Autodesk Inventor part; units mm, degrees
ref_plane "YZ Plane" through (0, 0, 0) normal (1, 0, 0) x (0, 1, 0)
ref_plane "XZ Plane" through (0, 0, 0) normal (0, 1, 0) x (-1, 0, 0)
ref_plane "XY Plane" through (0, 0, 0) normal (0, 0, 1) x (1, 0, 0)
sketch "Эскиз1" plane through (0, 0, 0) normal (0, 0, 1) x (1, 0, 0)
  line L0 (0, 0) -> (0, -10)
  line L1 (0, -10) -> (4, -10)
  line L2 (4, -10) -> (4, -26)
  line L3 (4, -26) -> (0, -26)
  line L4 (0, -26) -> (0, -29.9118)
  line L5 (0, -29.9118) -> (-1, -29.9118)
  arc A0 (-1, -29.9118) -> (-26.9172, -1) centre (-40, -38.8) ccw
  line L6 (-26.9172, -1) -> (-26.9172, 0)
  line L7 (-26.9172, 0) -> (-26, 0)
  line L8 (-26, 0) -> (-26, 4)
  line L9 (-26, 4) -> (-10, 4)
  line L10 (-10, 4) -> (-10, 0)
  line L11 (-10, 0) -> (0, 0)
  dimension "d0" = 40
  dimension "d1" = 1
  dimension "d3" = 38.8
  dimension "d4" = 4
  dimension "d5" = 40
  dimension "d6" = 16
  dimension "d7" = 10
  dimension "d8" = 16
  dimension "d9" = 10
extrude "Выдавливание1" add sketch "Эскиз1" along normal blind 4
properties part number "protector" material "Дерево (береза)"
Model file for the job. Use its own axes, mm. A direction names the side the tool comes from. Coordinates: 2 decimals unless noted, no trailing zeros. Order: outer loops, then holes, each group sorted by start corner. A loop starts at its lowest first (then second) coordinate and runs counter-clockwise, first axis right, second up. Notation, with made-up numbers: M -26.5,21.25 L 25.5,21.25 A14 cw 25.5,30.25 Z; hole C 60.25,79.5 d2. An arc over 180 degrees is marked long. Return JSON: item names as keys, results as strings.
1. Saw through at C-C (y = -7.5). Give the cut face in (x, z), and give its area (3 significant figures).
Ans:
{"outline": "M -15.09,0 L 0,0 L 0,4 L -15.09,4 Z", "area": "60.4 mm^2"}
2. Drill centre lines: probe 1 along X at (y, z) = (-0.5, 0.5); probe 2 along X at (y, z) = (2.5, 3.15); probe 3 along Y at (x, z) = (-22.5, 3.3). Where is each one in solid material? Low to high.
Ans:
{"probe 1": "-26.92 to 0", "probe 2": "-26 to -10", "probe 3": "-2.83 to 4"}
3. Tool access for faces 1 (the face through (-0.5, -29.912, 2)), 2 (the face through (2, -26, 2)), 3 (the face through (-10, 2, 2)), 4 (the face through (-26, 2, 2)): list every direction of +Z, -Z, +X, -X, +Y, -Y with a clear straight run to the whole face (end or side of a thin tool).
Ans:
{"face 1": "+Z, -Z, +X, -X, -Y", "face 2": "+Z, -Z, +X, -Y", "face 3": "+Z, -Z, +X, +Y", "face 4": "+Z, -Z, -X, +Y"}
4. Saw through at A-A (z = 0.8). Give the cut face in (x, y), and give its area (3 significant figures).
Ans:
{"outline": "M -26.92,-1 A40 cw -1,-29.91 L 0,-29.91 L 0,-26 L 4,-26 L 4,-10 L 0,-10 L 0,0 L -10,0 L -10,4 L -26,4 L -26,0 L -26.92,0 Z", "area": "427 mm^2"}
5. Flat gauge pins, fed straight in: pin 1 (1 mm diameter, centred on x = -12, y = -5.5, fed in from -Z); pin 2 (1.2 mm diameter, centred on y = 1, z = 3, fed in from +X); pin 3 (1.2 mm diameter, centred on y = -29, z = 1.5, fed in from +X); pin 4 (1.2 mm diameter, centred on y = 2, z = 2.5, fed in from -X). Where does each tip first touch, or does it go through?
Ans:
{"pin 1": "z = 0", "pin 2": "x = -10", "pin 3": "x = 0", "pin 4": "x = -26"}
6. Saw through at B-B (x = -2). Give the cut face in (y, z).
Ans:
{"outline": "M -26.31,0 L 0,0 L 0,4 L -26.31,4 Z"}
